```python
from build123d import *

# Parameters (mm, degrees)
F2_W     = 803
F2_H     = 735
F2_R     = 10
F2_R_2   = 301
F3_DEPTH = 3
F4_W     = 693
F4_H     = 10
F4_W_2   = 10
F4_H_2   = 735
F5_DEPTH = 50
F6_R     = 15
F6_R_2   = 10
F7_DEPTH = 50


with BuildPart() as f1:
    # F0 (on Front) → F1 (revolve)
    with BuildSketch(Plane.XZ):
        Polygon((-350, 3), (-300, 3), (-300, 55), (-301, 55), (-301, 95), (-349, 95), (-349, 55), (-350, 55), align=None)
        Polygon((-10, 3), (-300, 3), (-350, 3), (-350, 0), (-10, 0), align=None)
    revolve(axis=Axis((0, 0, 187.921241), (0, 0, -1)))

    # F2 (on Top) → F3 (join)
    with BuildSketch(Plane.XY):
        Rectangle(F2_W, F2_H)
        with Locations((-371.5, -337.5)):
            Circle(F2_R, mode=Mode.SUBTRACT)
        with Locations((371.5, -337.5)):
            Circle(F2_R, mode=Mode.SUBTRACT)
        Circle(F2_R_2, mode=Mode.SUBTRACT)
        with Locations((-371.5, 337.5)):
            Circle(F2_R, mode=Mode.SUBTRACT)
        with Locations((371.5, 337.5)):
            Circle(F2_R, mode=Mode.SUBTRACT)
    extrude(amount=F3_DEPTH)

    # F4 (on face) → F5 (join)
    with BuildSketch(Plane.XY.offset(3)):
        with Locations((0, -372.5)):
            Rectangle(F4_W, F4_H)
        with Locations((-396.5, 0)):
            Rectangle(F4_W_2, F4_H_2)
        with Locations((0, 372.5)):
            Rectangle(F4_W, F4_H)
        with Locations((396.5, 0)):
            Rectangle(F4_W_2, F4_H_2)
    extrude(amount=-F5_DEPTH)

    # F6 (on face) → F7 (join)
    with BuildSketch(Plane(origin=(0, 0, 0), x_dir=(1, 0, 0), z_dir=(0, 0, -1))):
        Circle(F6_R)
        Circle(F6_R_2, mode=Mode.SUBTRACT)
    extrude(amount=F7_DEPTH)


solid = f1.part
```
The model under review builds one solid part; all positions refer to its coordinate system, in mm. A direction names the side the tool comes from. Round coordinates to 2 decimals unless told otherwise and drop trailing zeros. Loops run counter-clockwise (first coordinate to the right, second up) from the corner with the lowest first, then second, coordinate; pieces in that order, holes last. Notation, with made-up numbers: (-10, -30.5) - (26, -30.5) arc R23 ccw to (26, -9.5) - close; hole circle Ø6 at (53.25, -1). An arc over 180 degrees is marked (long way). Use a Markdown table: item, result. Add a question column.
Q1. Add section C-C (x = -371.5). State the section outline as (y, z) points, plus the area to 4 significant figures.
Q2. Machinability: for faces 4 (the face through (392, 367.5, -17)), 5 (the face through (-391.5, -5, -23)), 6 (the face through (257.96, 236.55, 28.64)), 7 (the face through (-5, 367.5, -23)), which of the approach directions +Z, -Z, +X, -X, +Y, -Y give a long, thin tool a straight path to every point of the face, cutting with its end or side? Answer none if there is none.
Q3. For probe 1 along Y at (x, z) = (-371.5, 2.1); probe 2 along X at (y, z) = (337, 1); probe 3 along Y at (x, z) = (0, -34), list the stretches that pass through material, from the lowest coordinate up.
Q4. Insertion check: pin 1 Ø3 at (x, y) = (-395.5, 66) entering from -Z; pin 2 Ø10 at (x, z) = (153.5, 19) entering from -Y; pin 3 Ø16 at (x, y) = (371.5, -337.5) entering from -Z; pin 4 Ø3 at (x, z) = (292, 65.5) entering from -Y. Each pin has a flat end and moves straight along its axis. Give the tip position at first contact, or say it passes through.
Q5. Add section D-D (z = 84). State the section outline as (x, y) points.
Q6. The part is to be moulded in two halves that separate along Y. For faces 1 (the face through (221.85, 203.43, 75.28)), 2 (the face through (-392, -367.5, -17)), 3 (the face through (-5, 377.5, -22)), say which applies: pulls with the +Y half, pulls with the -Y half, needs draft (parallel to the pull), parting line crosses it, or undercut.
Worked answers:
| question | item | result |
|---|---|---|
| 1 | outline | (-367.5, 0) - (-347.5, 0) - (-347.5, 3) - (-367.5, 3) - close; (-327.5, 0) - (327.5, 0) - (327.5, 3) - (-327.5, 3) - close; (347.5, 0) - (367.5, 0) - (367.5, 3) - (347.5, 3) - close |
| 1 | area | 2,085 mm² |
| 2 | face 4 | +Z, -Z, +X, +Y |
| 2 | face 5 | -Z, +Y, -Y |
| 2 | face 6 | +Z |
| 2 | face 7 | -Z |
| 3 | probe 1 | -367.5 to -347.5, -327.5 to 327.5, 347.5 to 367.5 |
| 3 | probe 2 | -401.5 to -381.49, -361.51 to 361.51, 381.49 to 401.5 |
| 3 | probe 3 | -377.5 to -367.5, -15 to -10, 10 to 15, 367.5 to 377.5 |
| 4 | pin 1 | z = -47 |
| 4 | pin 2 | y = -316.93 |
| 4 | pin 3 | through |
| 4 | pin 4 | y = -193.42 |
| 5 | outline | circle Ø698 at (0, 0); hole circle Ø602 at (0, 0) |
| 6 | face 1 | undercut |
| 6 | face 2 | pulls with the -Y half |
| 6 | face 3 | pulls with the +Y half |
